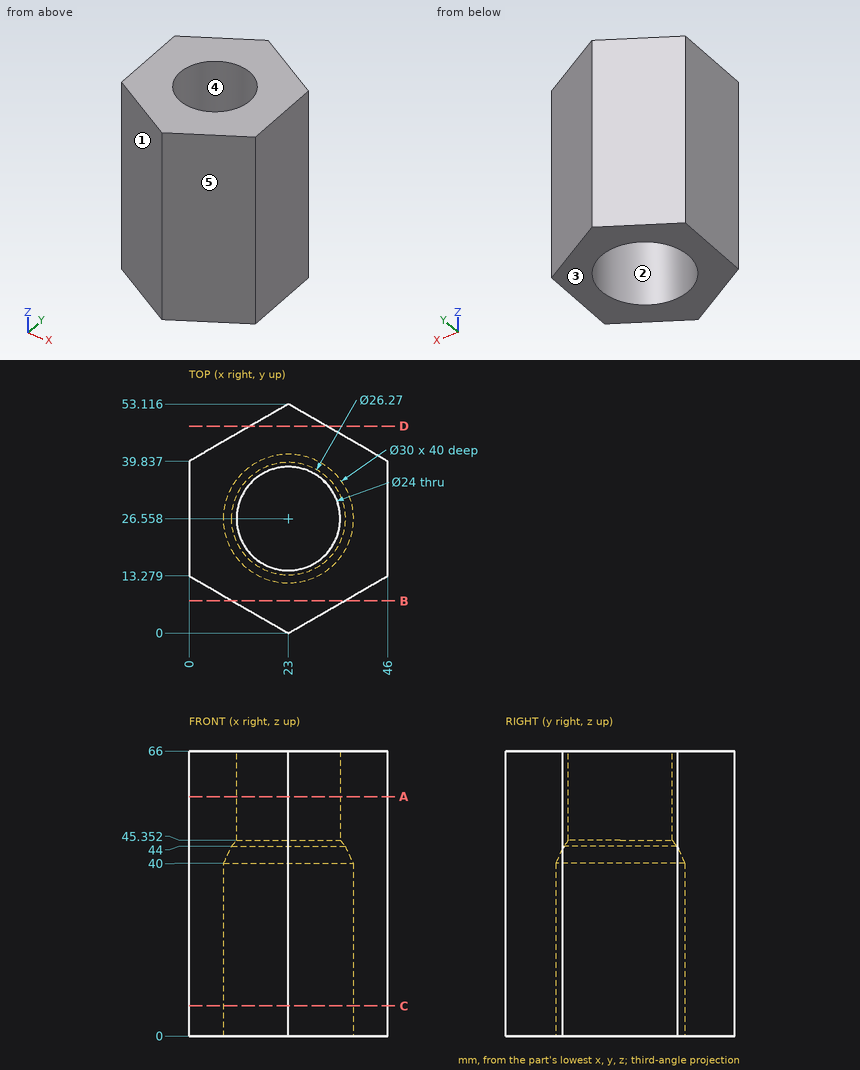
The drawing under review shows one solid part. Ordinate dimensions are in mm from its lowest x, y, z. A direction names the side the tool comes from. Give positions to 0.01 mm unless a question says otherwise; leave off trailing zeros. Write each loop counter-clockwise with the first axis right and the second up, starting at its lowest first coordinate (ties: lowest second). Pieces come first, ordered by that corner, then holes. Notation, with made-up numbers: (20.5, 10.25) - (67.5, 10.25) arc R21 ccw to (67.5, 48.25) - close; hole circle Ø10 at (23.25, -26.5). An arc over 180 degrees is marked (long way). Answer in a Markdown table with one row per item. Add a question column.
1. Insertion check: P1, Ø12, axis at x = 7.5, z = 15, coming from the +Y side; P2, Ø2, axis at x = 36.5, z = 31.5, coming from the -Y side; P3, Ø3, axis at y = 44.5, z = 36.5, coming from the +X side. Each pin has a flat end and moves straight along its axis. Give the tip position at first contact, or say it passes through.
2. We need section B-B on y = 7.5. Write out the cut boundary in (x, z), then the cut area to 3 significant figures.
3. Wall thickness on line 1 along Y through (x, z) = (23, 22.5) (1 decimal); line 2 along Y through (x, z) = (23, 50) (1 decimal); line 3 along X through (y, z) = (19, 27.5) (1 decimal): over which ranges is each line inside the solid? List them lowest first. Write a range as [from, to].
4. Draft analysis for pull direction Y (two halves, no side actions). For the marked faces 3, 4 and 5, state which applies: +Y half, -Y half, draft (parallel to the pull), parting line (faces both ways), or undercut.
5. We need section D-D on y = 48. Write out the cut boundary in (x, z).
6. We need section A-A on z = 55.5. Write out the cut boundary in (x, y), then the cut area to 3 significant figures.
7. We need section C-C on z = 7. Write out the cut boundary in (x, y).
8. Tool access review of the marked faces 1 and 2: name each direction out of +Z, -Z, +X, -X, +Y, -Y from which nothing blocks a thin tool from reaching the whole face with its end or side.
Ans:
| question | item | result |
|---|---|---|
| 1 | P1 | stops at y = 47.63 |
| 1 | P2 | stops at y = 7.22 |
| 1 | P3 | stops at x = 40.52 |
| 2 | outline | (10.01, 0) - (35.99, 0) - (35.99, 66) - (10.01, 66) - close |
| 2 | area | 1,710 mm^2 |
| 3 | line 1 | y = [0, 11.6], [41.6, 53.1] |
| 3 | line 2 | y = [0, 14.6], [38.6, 53.1] |
| 3 | line 3 | x = [0, 10], [36, 46] |
| 4 | face 3 | draft |
| 4 | face 4 | undercut |
| 4 | face 5 | -Y half |
| 5 | outline | (14.14, 0) - (31.86, 0) - (31.86, 66) - (14.14, 66) - close |
| 6 | outline | (0, 13.28) - (23, 0) - (46, 13.28) - (46, 39.84) - (23, 53.12) - (0, 39.84) - close; hole circle Ø24 at (23, 26.56) |
| 6 | area | 1,380 mm^2 |
| 7 | outline | (0, 13.28) - (23, 0) - (46, 13.28) - (46, 39.84) - (23, 53.12) - (0, 39.84) - close; hole circle Ø30 at (23, 26.56) |
| 8 | face 1 | +Z, -Z, -X, -Y |
| 8 | face 2 | -Z |
